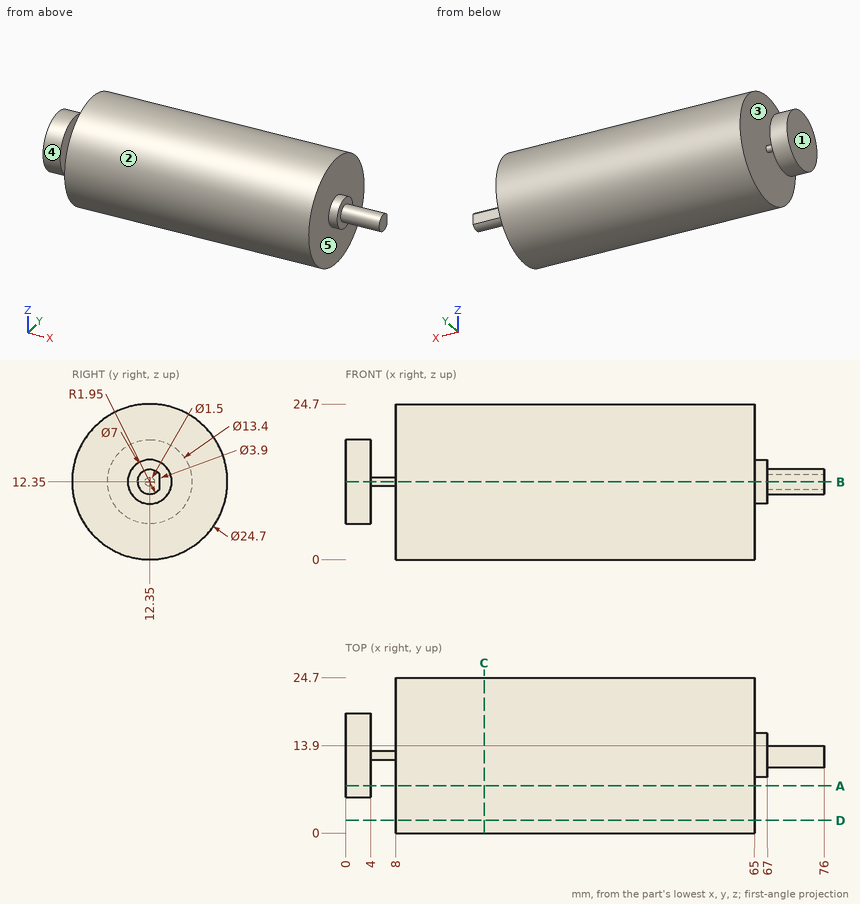
Check sheet for the drawn part. Datum: minimum x, y, z corner. Units: mm. A direction names the side the tool comes from. Coordinates: 2 decimals unless noted, no trailing zeros. Order: outer loops, then holes, each group sorted by start corner. A loop starts at its lowest first (then second) coordinate and runs counter-clockwise, first axis right, second up. Notation, with made-up numbers: M 30.5,26.5 L 63.5,26.5 A27 cw 63.5,61.5 Z; hole C 72,89.25 d3. An arc over 180 degrees is marked long. One line per question, with ' | ' between items. Start each with the question number.
Item 1: Material ranges on L1, parallel to X at y = 16.5, z = 11.5; L2, parallel to X at y = 17.75, z = 17; L3, parallel to Y at x = 39.5, z = 12.75, recorded low to high. Write a range as [from, to].
Item 2: Cross-section at B-B on z = 12.35. Enter the section's corners in (x, y).
Item 3: Gauge pin test, flat ends, axial feed: pin 1 (1.9 mm diameter, centred on x = 73.5, z = 13, fed in from +Y); pin 2 (1.5 mm diameter, centred on y = 6.5, z = 21, fed in from -X); pin 3 (6 mm diameter, centred on x = 27, z = 21, fed in from -Y). Record the tip position at first contact, or that the pin passes through.
Item 4: Set-up check for the marked faces 4 and 5: record each of +Z, -Z, +X, -X, +Y, -Y from which the full face is reachable in a straight line by a thin tool's end or side.
Item 5: Cross-section at A-A on y = 7.5. Enter the section's corners in (x, z).
Item 6: Cross-section at D-D on y = 2. Enter the section's corners in (x, z).
Item 7: Cross-section at C-C on x = 22. Enter the section's corners in (y, z).
Item 8: Draft check along X on the marked faces 1, 2 and 3. Enter one of: pulls with the +X half, pulls with the -X half, needs draft (parallel to the pull), parting line crosses it, or undercut.
Findings:
1) L1: x = [0, 4], [8, 65] | L2: x = [8, 65] | L3: y = [0.01, 24.69]
2) outline: M 0,5.65 L 4,5.65 L 4,11.6 L 8,11.6 L 8,0 L 65,0 L 65,8.85 L 67,8.85 L 67,10.4 L 76,10.4 L 76,13.9 L 67,13.9 L 67,15.85 L 65,15.85 L 65,24.7 L 8,24.7 L 8,13.1 L 4,13.1 L 4,19.05 L 0,19.05 Z
3) pin 1: stops at y = 13.9 | pin 2: stops at x = 8 | pin 3: stops at y = 1.37
4) face 4: -X | face 5: +X
5) outline: M 0,7.73 L 4,7.73 L 4,16.97 L 0,16.97 Z; M 8,0.99 L 65,0.99 L 65,23.71 L 8,23.71 Z
6) outline: M 8,5.61 L 65,5.61 L 65,19.09 L 8,19.09 Z
7) outline: C 12.35,12.35 d24.7
8) face 1: pulls with the -X half | face 2: needs draft | face 3: undercut
